Geometry: final body of the model. Coordinates: model frame, mm. Give positions to 0.01 mm unless a question says otherwise; leave off trailing zeros. Loops run counter-clockwise (first coordinate to the right, second up) from the corner with the lowest first, then second, coordinate; pieces in that order, holes last. Notation, with made-up numbers: (13.5, 32) -> (45.5, 32) arc R25 ccw to (45.5, 63) -> close; hole circle Ø1 at (46.5, 84.25). An arc over 180 degrees is marked (long way). One line per question, with ' | ' between items. Start each with the question number.
Item 1: Section D-D on y = -2.75. Return loops of the section in (x, z).
Item 2: Material intervals for line 1 along Z through (x, y) = (4, -0.25); line 2 along Z through (x, y) = (-3, -3); line 3 along X through (y, z) = (-3, 2), sorted ascending. Write a range as [from, to].
Item 3: Section C-C on z = 2.75. Return loops of the section in (x, y).
Item 4: Pin query (flat end, axial travel): P1, Ø0.7, axis at x = 5, z = 0.5, coming from the -Y side; P2, Ø2, axis at x = 1.5, y = -1, coming from the +Z side; P3, Ø2, axis at y = 1, z = -2.5, coming from the -X side. Return the tip coordinate at first contact, or that it passes through.
Item 5: Mould query, pull axis X, two halves, no side actions, for faces 1 (the flat face through (3, 0, 3.7)), 2 (the cylindrical face through (-4.596, 0.197, 0.345)), 3 (the flat face through (0, 0, 3.69)). Classes: released by +X, released by -X, zero draft, split by the parting line, or undercut.
from build123d import *

# Parameters (mm, degrees)
EXTRUDE_1_DEPTH     = 0.7
SKETCH_2_R          = 4.05
EXTRUDE_2_DEPTH     = 3
SKETCH_3_W          = 5.2
SKETCH_3_H          = 4.2
CUT_EXTRUDE_1_DEPTH = 0.01
SKETCH_4_R          = 0.25
EXTRUDE_3_DEPTH     = 4


with BuildPart() as part:
    # Эскиз1 → Бобышка-Вытянуть1 (new body)
    with BuildSketch(Plane.XY):
        with BuildLine():
            Line((5.2, 0.4), (4.582575695, 0.4))
            ThreePointArc((4.582575695, 0.4), (-4.6, 0), (4.582575695, -0.4))
            Line((4.582575695, -0.4), (5.2, -0.4))
            ThreePointArc((5.2, -0.4), (5.6, 0), (5.2, 0.4))
        make_face()
    extrude(amount=EXTRUDE_1_DEPTH)

    # Эскиз2 → Бобышка-Вытянуть2 (add)
    with BuildSketch(Plane.XY.offset(0.7)):
        Circle(SKETCH_2_R)
    extrude(amount=EXTRUDE_2_DEPTH)

    # Эскиз3 → Вырез-Вытянуть1 (cut)
    with BuildSketch(Plane.XY.offset(3.7)):
        Rectangle(SKETCH_3_W, SKETCH_3_H)
    extrude(amount=-CUT_EXTRUDE_1_DEPTH, mode=Mode.SUBTRACT)

    # Эскиз4 → Бобышка-Вытянуть3 (add)
    with BuildSketch(Plane.XY):
        with Locations((1.796, -1.796)):
            Circle(SKETCH_4_R)
        with Locations((1.796, 1.796)):
            Circle(SKETCH_4_R)
        with Locations((-1.796, 1.796)):
            Circle(SKETCH_4_R)
        with Locations((-1.796, -1.796)):
            Circle(SKETCH_4_R)
    extrude(amount=-EXTRUDE_3_DEPTH)


solid = part.part
Result sheet:
1) outline: (-3.69, 0) -> (3.69, 0) -> (3.69, 0.7) -> (2.97, 0.7) -> (2.97, 3.7) -> (-2.97, 3.7) -> (-2.97, 0.7) -> (-3.69, 0.7) -> close
2) line 1: z = [0, 3.7] | line 2: z = [0, 0.7] | line 3: x = [-2.72, 2.72]
3) outline: circle Ø8.1 at (0, 0)
4) P1: stops at y = -0.4 | P2: stops at z = 3.69 | P3: stops at x = -2.05
5) face 1: zero draft | face 2: split by the parting line | face 3: undercut
